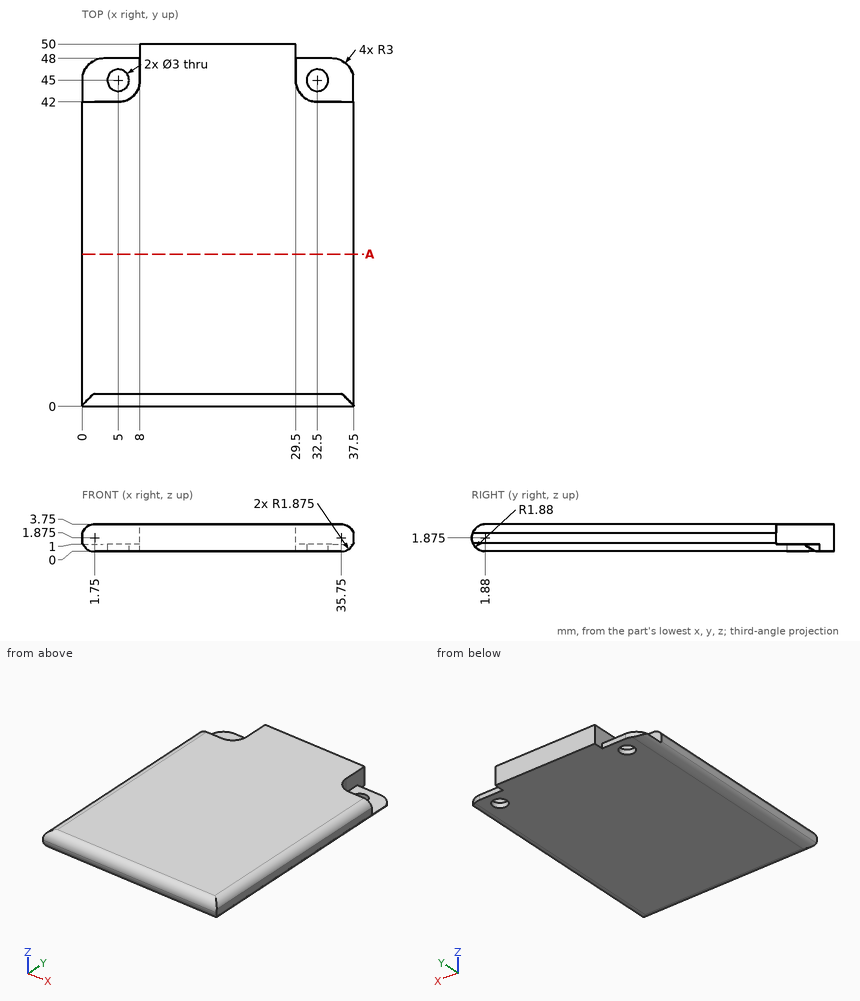
Print and shaded views of the part. All mm, measured from the part's lowest x, y and z. Give positions to 0.01 mm unless a question says otherwise; leave off trailing zeros. Write each loop counter-clockwise with the first axis right and the second up, starting at its lowest first coordinate (ties: lowest second). Pieces come first, ordered by that corner, then holes. Notation, with made-up numbers: (60.5, 74.5) -> (65.5, 74.5) arc R29 ccw to (65.5, 99.5) -> close; hole circle Ø4 at (13.25, 3). An arc over 180 degrees is marked (long way). Use CSV: the item, a comma, the result in double quotes. Start each with the question number.
1) Pin check, flat tips, straight feed: P1, Ø1.9, axis at y = 47.5, z = 2.5, coming from the -X side; P2, Ø3, axis at x = 4.5, y = 44.5, coming from the +Z side; P3, Ø0.8, axis at x = 2.5, z = 2.5, coming from the +Y side. Stop position of each tip, or through.
2) Drill centre lines: L1, parallel to Y at x = 32.5, z = 0.7; L2, parallel to Y at x = 5, z = 0.35; L3, parallel to Y at x = 11.5, z = 3.25. Where is each one in solid material? Low to high.
3) Cut at A-A on y = 21. List the corners of the cut face in (x, z) (3 decimals).
Final values:
1,P1,"stops at x = 8"
1,P2,"stops at z = 1"
1,P3,"stops at y = 42"
2,L1,"y = 0.41 to 43.5, 46.5 to 48"
2,L2,"y = 0.78 to 43.5, 46.5 to 48"
2,L3,"y = 0.6 to 50"
3,outline,"(0, 1.202) arc R1.875 ccw to (1.75, 0) -> (35.75, 0) arc R1.875 ccw to (37.5, 1.202) -> (37.5, 2.548) arc R1.875 ccw to (35.75, 3.75) -> (1.75, 3.75) arc R1.875 ccw to (0, 2.548) -> close"
